CAD build for the part. Positions are in the model's coordinates, mm. Face numbers are marked on the shaded views. A direction names the side the tool comes from. Give positions to 0.01 mm unless a question says otherwise; leave off trailing zeros. Loops run counter-clockwise (first coordinate to the right, second up) from the corner with the lowest first, then second, coordinate; pieces in that order, holes last.
```python
from build123d import *

# Parameters (mm, degrees)
SKETCH1_W           = 22
SKETCH1_H           = 72
BOSS_EXTRUDE2_DEPTH = 5
SKETCH2_W           = 14
SKETCH2_H           = 30
CUT_EXTRUDE1_DEPTH  = 38.973675092
SKETCH3_W           = 3
SKETCH3_H           = 5
CUT_EXTRUDE2_DEPTH  = 38.973675092
SKETCH4_R           = 1.5
CUT_EXTRUDE3_DEPTH  = 38.973675092
SKETCH5_W           = 7.5
SKETCH5_H           = 15
BOSS_EXTRUDE3_DEPTH = 20
CHAMFER2_SIZE       = 5
SKETCH6_W           = 7
SKETCH6_H           = 15
CUT_EXTRUDE4_DEPTH  = 43.626282972
SKETCH7_W           = 8
SKETCH7_H           = 5
CUT_EXTRUDE5_DEPTH  = 2
CHAMFER6_SIZE       = 5
FILLET3_R           = 1
FILLET6_R           = 10
SKETCH9_R           = 2.38125
CUT_EXTRUDE6_DEPTH  = 50.040799341
CHAMFER8_SIZE       = 1


with BuildPart() as part:
    # Sketch1 → Boss-Extrude2 (new body)
    with BuildSketch(Plane(origin=(0, 0, 0), x_dir=(1, 0, 0), z_dir=(0, 1, 0))):
        Rectangle(SKETCH1_W, SKETCH1_H)
    extrude(amount=BOSS_EXTRUDE2_DEPTH)

    # Sketch2 → Cut-Extrude1 (cut, through all)
    with BuildSketch(Plane(origin=(0, 5, 0), x_dir=(1, 0, 0), z_dir=(0, 1, 0))):
        with Locations((0, 9)):
            Rectangle(SKETCH2_W, SKETCH2_H)
    extrude(amount=-CUT_EXTRUDE1_DEPTH, mode=Mode.SUBTRACT)

    # Sketch3 → Cut-Extrude2 (cut, through all)
    with BuildSketch(Plane(origin=(0, 5, 0), x_dir=(1, 0, 0), z_dir=(0, 1, 0))):
        with Locations((-5.5, 26.5)):
            Rectangle(SKETCH3_W, SKETCH3_H)
        with Locations((5.5, 26.5)):
            Rectangle(SKETCH3_W, SKETCH3_H)
        with Locations((-5.5, -8.5)):
            Rectangle(SKETCH3_W, SKETCH3_H)
        with Locations((5.5, -8.5)):
            Rectangle(SKETCH3_W, SKETCH3_H)
    extrude(amount=-CUT_EXTRUDE2_DEPTH, mode=Mode.SUBTRACT)

    # Sketch4 → Cut-Extrude3 (cut, through all)
    with BuildSketch(Plane(origin=(0, 5, 0), x_dir=(1, 0, 0), z_dir=(0, 1, 0))):
        with Locations(Location((0, 26.5, 0), (0, 0, 270))):
            Circle(SKETCH4_R)
        with Locations(Location((0, -8.5, 0), (0, 0, 270))):
            Circle(SKETCH4_R)
    extrude(amount=-CUT_EXTRUDE3_DEPTH, mode=Mode.SUBTRACT)

    # Sketch5 → Boss-Extrude3 (add)
    with BuildSketch(Plane(origin=(0, 5, 0), x_dir=(1, 0, 0), z_dir=(0, 1, 0))):
        with Locations((-7.25, -28.5)):
            Rectangle(SKETCH5_W, SKETCH5_H)
    boss_extrude3 = extrude(amount=BOSS_EXTRUDE3_DEPTH)

    # Mirror1: Boss-Extrude3 across plane
    add(boss_extrude3.mirror(Plane(origin=(0, 0, 0), x_dir=(0, 0, 1), z_dir=(1, 0, 0))))

    # Chamfer2
    chamfer2_edges = [part.edges().sort_by_distance(p)[0] for p in [
        (0, 0, 36),
    ]]
    chamfer(chamfer2_edges, length=CHAMFER2_SIZE - 0.0001)  # a hair under: the kernel refuses the full size

    # Sketch6 → Cut-Extrude4 (cut, through all)
    with BuildSketch(Plane(origin=(0, 5, 0), x_dir=(1, 0, 0), z_dir=(0, 1, 0))):
        with Locations((0, -28.5)):
            Rectangle(SKETCH6_W, SKETCH6_H)
    extrude(amount=-CUT_EXTRUDE4_DEPTH, mode=Mode.SUBTRACT)

    # Sketch7 → Cut-Extrude5 (cut)
    with BuildSketch(Plane(origin=(0, 5, 0), x_dir=(1, 0, 0), z_dir=(0, 1, 0))):
        with Locations((0, 26.5)):
            Rectangle(SKETCH7_W, SKETCH7_H)
        with Locations((0, -8.5)):
            Rectangle(SKETCH7_W, SKETCH7_H)
    extrude(amount=-CUT_EXTRUDE5_DEPTH, mode=Mode.SUBTRACT)

    # Chamfer6
    chamfer6_edges = [part.edges().sort_by_distance(p)[0] for p in [
        (-11, 2.5, -36),
        (11, 2.5, -36),
    ]]
    chamfer(chamfer6_edges, length=CHAMFER6_SIZE)

    # Fillet3
    fillet3_edges = [part.edges().sort_by_distance(p)[0] for p in [
        (-7, 2.5, -29),
        (-4, 1.5, -29),
        (-4, 1.5, -24),
        (7, 2.5, -29),
        (4, 1.5, -24),
        (4, 1.5, -29),
        (-7, 2.5, 11),
        (-4, 1.5, 6),
        (-4, 1.5, 11),
        (7, 2.5, 11),
        (4, 1.5, 11),
        (4, 1.5, 6),
    ]]
    fillet(fillet3_edges, radius=FILLET3_R)

    # Fillet6
    fillet6_edges = [part.edges().sort_by_distance(p)[0] for p in [
        (-7.25, 5, 21),
        (7.25, 5, 21),
    ]]
    fillet(fillet6_edges, radius=FILLET6_R - 0.0001)  # a hair under: the kernel refuses the full size

    # Sketch9 → Cut-Extrude6 (cut, through all)
    with BuildSketch(Plane.ZY.offset(11)):
        with Locations((28.5, 20)):
            Circle(SKETCH9_R)
        with Locations((28.5, 10)):
            Circle(SKETCH9_R)
    extrude(amount=-CUT_EXTRUDE6_DEPTH, mode=Mode.SUBTRACT)

    # Chamfer8
    chamfer8_edges = [part.edges().sort_by_distance(p)[0] for p in [
        (-7.25, 25, 36),
        (-7.25, 25, 21),
        (7.25, 25, 21),
        (7.25, 25, 36),
    ]]
    chamfer(chamfer8_edges, length=CHAMFER8_SIZE)


solid = part.part
```
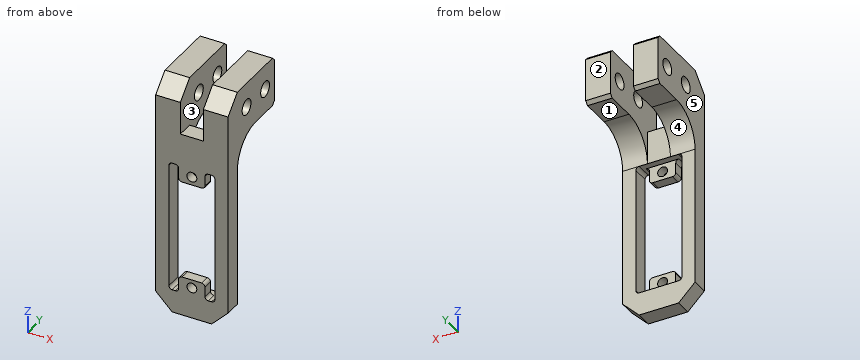
1. Saw through at A-A, the plane z = 8.5. List the corners of the cut face in (x, y).
Responses:
outline: (-11, 0) - (-7, 0) - (-7, 5) - (-11, 5) - close; (-4, 0) - (-1.5, 0) - (-1.5, 3) - (-4, 3) - close; (1.5, 0) - (4, 0) - (4, 3) - (1.5, 3) - close; (7, 0) - (11, 0) - (11, 5) - (7, 5) - close
2. Saw through at C-C, the plane x = 0. List the corners of the cut face in (y, z), and give its area (3 significant figures).
Responses:
outline: (0, -36) - (5, -36) - (5, -29) - (3, -29) - (3, -28) - (0, -28) - close; (0, -25) - (3, -25) - (3, -24) - (0, -24) - close; (0, 6) - (3, 6) - (3, 7) - (0, 7) - close; (0, 10) - (3, 10) - (3, 11) - (5, 11) - (5, 21) - (0, 21) - close
area: 97.0 mm2
3. Probe line 1 along Y through (x, z) = (8, 28.5); line 2 along X through (y, z) = (13, 30.5); line 3 along X through (y, z) = (4.5, -15.5). List the from-to ranges inside material, lowest first.
Responses:
line 1: y = 0 to 7.62, 12.38 to 17.62, 22.38 to 25
line 2: x = -11 to -3.5, 3.5 to 11
line 3: x = -11 to -7, 7 to 11
4. Tool access for the marked faces 1 and 2: list every direction of +Z, -Z, +X, -X, +Y, -Y with a clear straight run to the whole face (end or side of a thin tool).
Responses:
face 1: -Z, +X, -X, +Y
face 2: +Z, -Z, +X, -X, +Y
5. Pull direction X, two halves, no side cores. Call the marked faces 3, 4 and 5: released by +X, released by -X, zero draft, split by the parting line, or undercut.
Responses:
face 3: undercut
face 4: zero draft
face 5: released by -X
6. Saw through at D-D, the plane y = 20. List the corners of the cut face in (x, z), and give its area (3 significant figures).
Responses:
outline: (-11, 21) - (-3.5, 21) - (-3.5, 26.12) - (-11, 26.12) - close; (-11, 30.88) - (-3.5, 30.88) - (-3.5, 36) - (-11, 36) - close; (3.5, 21) - (11, 21) - (11, 26.12) - (3.5, 26.12) - close; (3.5, 30.88) - (11, 30.88) - (11, 36) - (3.5, 36) - close
area: 154 mm2
7. Saw through at B-B, the plane z = 28.5. List the corners of the cut face in (x, y), and give its area (3 significant figures).
Responses:
outline: (-11, 0) - (-3.5, 0) - (-3.5, 7.62) - (-11, 7.62) - close; (-11, 12.38) - (-3.5, 12.38) - (-3.5, 17.62) - (-11, 17.62) - close; (-11, 22.38) - (-3.5, 22.38) - (-3.5, 25) - (-11, 25) - close; (3.5, 0) - (11, 0) - (11, 7.62) - (3.5, 7.62) - close; (3.5, 12.38) - (11, 12.38) - (11, 17.62) - (3.5, 17.62) - close; (3.5, 22.38) - (11, 22.38) - (11, 25) - (3.5, 25) - close
area: 232 mm2
8. Drop flat-ended pins along their axis: pin 1 (5.5 mm diameter, centred on x = -2, z = 7.5, fed in from +Y); pin 2 (8 mm diameter, centred on x = 7, y = 19, fed in from -Z); pin 3 (2.5 mm diameter, centred on x = 3, y = 3, fed in from +Z); pin 4 (8 mm diameter, centred on x = 2.5, z = 4.5, fed in from -Y). Give the stop position or say it passes through.
Responses:
pin 1: stops at y = 3
pin 2: stops at z = 21
pin 3: stops at z = 35.15
pin 4: stops at y = 0
